Input: part model. Units: mm. Frame: model coordinates. A direction names the side the tool comes from. Round coordinates to 2 decimals unless told otherwise and drop trailing zeros. Order: outer loops, then holes, each group sorted by start corner. A loop starts at its lowest first (then second) coordinate and runs counter-clockwise, first axis right, second up. Notation, with made-up numbers: (10.5, 50) - (52.5, 50) arc R19 cw to (52.5, 62) - close; hole circle Ø7 at (-30.5, 66.25). An arc over 180 degrees is marked (long way). One line per item, written item: value. Start each with the question number.
from build123d import *

# Parameters (mm, degrees)
BOSS_EXTRUDE1_DEPTH                                 = 221.5
CSK_FOR_M3_COUNTERSUNK_FLAT_HEAD_SCREW1_D           = 3
CSK_FOR_M3_COUNTERSUNK_FLAT_HEAD_SCREW1_CSINK_D     = 5.5
CSK_FOR_M3_COUNTERSUNK_FLAT_HEAD_SCREW1_CSINK_ANGLE = 90
CSK_FOR_M3_COUNTERSUNK_FLAT_HEAD_SCREW4_D           = 3
CSK_FOR_M3_COUNTERSUNK_FLAT_HEAD_SCREW4_CSINK_D     = 5.5
CSK_FOR_M3_COUNTERSUNK_FLAT_HEAD_SCREW4_CSINK_ANGLE = 90
SKETCH12_W                                          = 8
SKETCH12_H                                          = 7
BOSS_EXTRUDE2_DEPTH                                 = 5.5
CUT_EXTRUDE1_DEPTH                                  = 359
BOSS_EXTRUDE3_DEPTH                                 = 3
BOSS_EXTRUDE4_DEPTH                                 = 2.5
BOSS_EXTRUDE4_DEPTH_BACK                            = 6
SKETCH19_W                                          = 9
SKETCH19_H                                          = 2
CUT_EXTRUDE2_DEPTH                                  = 10
SKETCH20_W                                          = 0.6
SKETCH20_H                                          = 225
CUT_EXTRUDE3_DEPTH                                  = 10
SKETCH22_W                                          = 0.6
SKETCH22_H                                          = 225
CUT_EXTRUDE4_DEPTH                                  = 10
SKETCH25_W                                          = 8.4
SKETCH25_H                                          = 5.5
CUT_EXTRUDE5_DEPTH                                  = 10
BOSS_EXTRUDE5_DEPTH                                 = 2
TAP_DRILL_FOR_M4X0_7_TAP1_D                         = 4
TAP_DRILL_FOR_M4X0_7_TAP1_DEPTH                     = 5
BOSS_EXTRUDE6_DEPTH                                 = 221.5
FILLET1_R                                           = 1


with BuildPart() as part:
    # Sketch1 → Boss-Extrude1 (new body)
    with BuildSketch(Plane(origin=(0, 0, 0), x_dir=(1, 0, 0), z_dir=(0, 1, 0))):
        Polygon((0, 0), (0, 9), (9, 9), (9, 7), (2, 7), (2, 0), align=None)
    extrude(amount=BOSS_EXTRUDE1_DEPTH)

    # CSK for M3 Countersunk Flat Head Screw1 (through all)
    with Locations(Plane.ZY):
        with Locations((-4, 211), (-4, 40.25)):
            CounterSinkHole(CSK_FOR_M3_COUNTERSUNK_FLAT_HEAD_SCREW1_D / 2, CSK_FOR_M3_COUNTERSUNK_FLAT_HEAD_SCREW1_CSINK_D / 2, counter_sink_angle=CSK_FOR_M3_COUNTERSUNK_FLAT_HEAD_SCREW1_CSINK_ANGLE)

    # CSK for M3 Countersunk Flat Head Screw4 (through all)
    with Locations(Plane(origin=(0, 0, -9), x_dir=(-1, 0, 0), z_dir=(0, 0, -1))):
        with Locations((-5, 120)):
            CounterSinkHole(CSK_FOR_M3_COUNTERSUNK_FLAT_HEAD_SCREW4_D / 2, CSK_FOR_M3_COUNTERSUNK_FLAT_HEAD_SCREW4_CSINK_D / 2, counter_sink_angle=CSK_FOR_M3_COUNTERSUNK_FLAT_HEAD_SCREW4_CSINK_ANGLE)

    # Sketch12 → Boss-Extrude2 (add)
    with BuildSketch(Plane.XZ):
        with Locations((5, -3.5)):
            Rectangle(SKETCH12_W, SKETCH12_H)
    extrude(amount=-BOSS_EXTRUDE2_DEPTH)

    # Sketch13 → Cut-Extrude1 (cut)
    with BuildSketch(Plane(origin=(0, 221.5, 0), x_dir=(1, 0, 0), z_dir=(0, 1, 0))):
        Polygon((0, 8), (1, 9), (0, 9), align=None)
    extrude(amount=-CUT_EXTRUDE1_DEPTH, mode=Mode.SUBTRACT)

    # Sketch14 → Boss-Extrude3 (add)
    with BuildSketch(Plane.XZ):
        Polygon((0, 0), (9, 0), (9, -9), (1, -9), (0, -8), align=None)
    extrude(amount=BOSS_EXTRUDE3_DEPTH)

    # Sketch18 → Boss-Extrude4 (add, two sides: drawn at the far end of the back side and taken through both)
    with BuildSketch(Plane(origin=(0, 221.5, 0), x_dir=(1, 0, 0), z_dir=(0, 1, 0)).offset(-BOSS_EXTRUDE4_DEPTH_BACK)):
        Polygon((0, 0), (9, 0), (9, 9), (1, 9), (0, 8), align=None)
    extrude(amount=BOSS_EXTRUDE4_DEPTH + BOSS_EXTRUDE4_DEPTH_BACK)

    # Sketch19 → Cut-Extrude2 (cut)
    with BuildSketch(Plane(origin=(0, 0, -9), x_dir=(-1, 0, 0), z_dir=(0, 0, -1))):
        with Locations((-4.5, 223)):
            Rectangle(SKETCH19_W, SKETCH19_H)
    extrude(amount=-CUT_EXTRUDE2_DEPTH, mode=Mode.SUBTRACT)

    # Sketch20 → Cut-Extrude3 (cut)
    with BuildSketch(Plane.ZY):
        with Locations((-0.3, 109.5)):
            Rectangle(SKETCH20_W, SKETCH20_H)
    extrude(amount=-CUT_EXTRUDE3_DEPTH, mode=Mode.SUBTRACT)

    # Sketch22 → Cut-Extrude4 (cut)
    with BuildSketch(Plane(origin=(0, 0, -9), x_dir=(-1, 0, 0), z_dir=(0, 0, -1))):
        with Locations((-8.7, 109.5)):
            Rectangle(SKETCH22_W, SKETCH22_H)
    extrude(amount=-CUT_EXTRUDE4_DEPTH, mode=Mode.SUBTRACT)

    # Sketch25 → Cut-Extrude5 (cut)
    with BuildSketch(Plane.ZY):
        with Locations((-4.8, -0.25)):
            Rectangle(SKETCH25_W, SKETCH25_H)
    extrude(amount=-CUT_EXTRUDE5_DEPTH, mode=Mode.SUBTRACT)

    # Sketch29 → Boss-Extrude5 (add)
    with BuildSketch(Plane.XZ.offset(-2.5)):
        Polygon((8.4, -0.6), (0, -0.6), (0, -8), (1, -9), (8.4, -9), align=None)
    extrude(amount=BOSS_EXTRUDE5_DEPTH)

    # Tap Drill for M4x0.7 Tap1
    with Locations(Plane(origin=(0, 0.5, 0), x_dir=(-1, 0, 0), z_dir=(0, -1, 0))):
        with Locations((-5.4, 3.6)):
            Hole(TAP_DRILL_FOR_M4X0_7_TAP1_D / 2, depth=TAP_DRILL_FOR_M4X0_7_TAP1_DEPTH)

    # Sketch32 → Boss-Extrude6 (add)
    with BuildSketch(Plane(origin=(0, 222, 0), x_dir=(1, 0, 0), z_dir=(0, 1, 0))):
        Polygon((1, 9), (0, 8), (0, 9), align=None)
    extrude(amount=-BOSS_EXTRUDE6_DEPTH)

    # Fillet1
    fillet1_edges = [part.edges().sort_by_distance(p)[0] for p in [
        (0, 111.25, -9),
    ]]
    fillet(fillet1_edges, radius=FILLET1_R)


solid = part.part
Item 1: Line query: L1, parallel to Y at x = 1.5, z = -4; L2, parallel to Y at x = 8.25, z = -1.25; L3, parallel to X at y = 120, z = -7.25. Output: solid intervals per line, ascending.
Item 2: Section query B-B on y = 156.5. Return loops of the section in (x, z), and give its area (3 significant figures).
Item 3: Section query A-A on x = 5. Return loops of the section in (y, z), and give its area (3 significant figures).
Item 4: Reachability of faces 1 (the face through (3.7, 5.5, -5.2)), 2 (the face through (1, 112, -0.6)) from +Z, -Z, +X, -X, +Y, -Y: full face, straight path, thin tool, end or side. Return the list, or none.
Item 5: Pull-direction query (Y, two-part tool) for faces 3 (the face through (2, 109, -4)), 4 (the face through (3.8, 3, -2.4)), 5 (the face through (4, 222, -5)); classes: released by +Y, released by -Y, zero draft, split by the parting line, or undercut.
Item 6: First-contact query: pin 1 Ø3.5 at (y, z) = (211, -4) entering from -X; pin 2 Ø4 at (y, z) = (75, -1.5) entering from +X; pin 3 Ø2.5 at (x, y) = (5, 120) entering from -Z; pin 4 Ø3 at (x, y) = (4, 61.5) entering from +Z. Flat tips, straight axial feed; report the tip coordinate or a pass-through.
Geometry results:
1. L1: y = 0.5 to 38.75, 41.75 to 209.5, 212.5 to 222
1. L2: y = 0.5 to 5.5, 215.5 to 222
1. L3: x = 0 to 3.5, 6.5 to 8.4
2. outline: (0, -8) arc R1 ccw to (1, -9) - (8.4, -9) - (8.4, -7) - (2, -7) - (2, -0.6) - (0, -0.6) - close
2. area: 29.4 mm^2
3. outline: (0.5, -9) - (117.25, -9) - (118.5, -7.75) - (118.5, -7) - (5.5, -7) - (5.5, -5.56) - (0.5, -5.56) - close; (0.5, -1.64) - (5.5, -1.64) - (5.5, -0.6) - (0.5, -0.6) - close; (121.5, -7.75) - (122.75, -9) - (222, -9) - (222, -0.6) - (215.5, -0.6) - (215.5, -7) - (121.5, -7) - close
3. area: 489 mm^2
4. face 1: +Z, +X
4. face 2: +Z, +X, -X, +Y, -Y
5. face 3: undercut
5. face 4: zero draft
5. face 5: released by +Y
6. pin 1: stops at x = 1
6. pin 2: stops at x = 2
6. pin 3: passes through
6. pin 4: stops at z = -7
